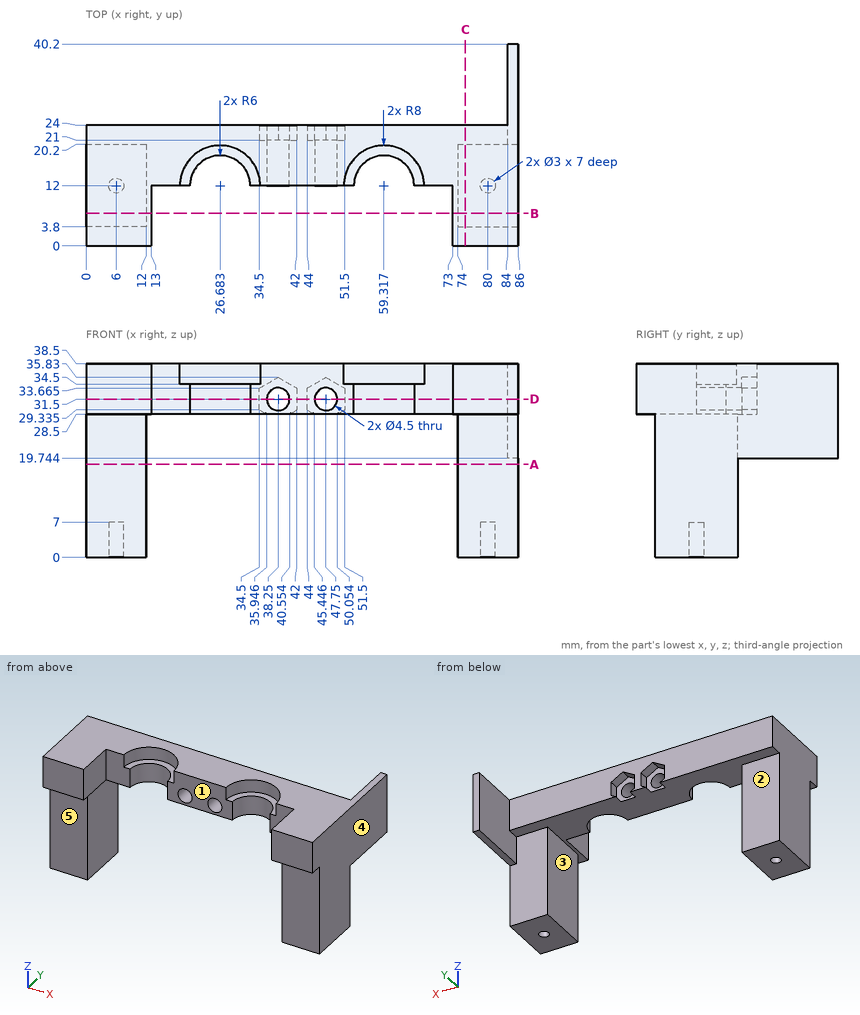
Verification items for this drawing (mm, ordinates from the low corner). A direction names the side the tool comes from. Coordinates: 2 decimals unless noted, no trailing zeros. Write each loop counter-clockwise with the first axis right and the second up, starting at its lowest first coordinate (ties: lowest second). Pieces come first, ordered by that corner, then holes. Notation, with made-up numbers: M -39,13 L -34,13 A24 ccw -34,37 Z; hole C 23,20 d11. An arc over 180 degrees is marked long. One line per item, written item: value. Start each with the question number.
(1) Scan lines: line 1 along X through (y, z) = (12, 2.5); line 2 along Y through (x, z) = (6, 4); line 3 along Z through (x, y) = (38.25, 15.75). Record each from-to range of solid material in increasing order. Write a range as [from, to].
(2) Sectioned sample at B-B, the plane y = 6.5. Enter the section's corners in (x, z), and give its area (3 significant figures).
(3) Sectioned sample at C-C, the plane x = 75.5. Enter the section's corners in (y, z).
(4) Tool access check on the marked faces 1, 2, 3, 4 and 5. Record the directions out of +Z, -Z, +X, -X, +Y, -Y that give a thin tool (end or side, any length) a straight path to the whole face; none if there is none.
(5) Sectioned sample at A-A, the plane z = 18.5. Enter the section's corners in (x, y).
(6) Sectioned sample at D-D, the plane z = 31.5. State how many separate pieces and enclosed holes the cut face has, and give its area (3 significant figures).
(7) Depth check by flat-ended pin: pin 1 (3 mm diameter, centred on x = 28, z = 33, fed in from +Y); pin 2 (9.5 mm diameter, centred on x = 82, z = 19, fed in from -Y); pin 3 (11 mm diameter, centred on x = 38, z = 33.5, fed in from -Y). Enter the tip coordinate at first touch or a pass-through.
Filled sheet:
1. line 1: [0, 4.5], [7.5, 12], [74, 78.5], [81.5, 86]
1. line 2: [3.8, 10.5], [13.5, 20.2]
1. line 3: [28.5, 29.25], [33.75, 38.5]
2. outline: M 0,0 L 12,0 L 12,28.5 L 13,28.5 L 13,38.5 L 0,38.5 Z; M 73,28.5 L 74,28.5 L 74,0 L 86,0 L 86,38.5 L 73,38.5 Z
2. area: 944 mm²
3. outline: M 0,28.5 L 3.8,28.5 L 3.8,0 L 20.2,0 L 20.2,28.5 L 24,28.5 L 24,38.5 L 0,38.5 Z
4. face 1: +Z, -Z, -Y
4. face 2: -Z, -X, +Y
4. face 3: -Z, +Y, -Y
4. face 4: +Z, -Z, +X, +Y, -Y
4. face 5: -Z, +X, -X, -Y
5. outline: M 0,3.8 L 12,3.8 L 12,20.2 L 0,20.2 Z; M 74,3.8 L 86,3.8 L 86,20.2 L 74,20.2 Z
6. separate pieces: 3
6. enclosed holes: 0
6. area: 1,140 mm²
7. pin 1: y = 24
7. pin 2: y = 3.8
7. pin 3: y = 12
